Source: CAD feature listing. Evaluate the final solid. Frame: model axes, mm. Face numbers are marked on the shaded views. A direction names the side the tool comes from. Give positions to 0.01 mm unless a question says otherwise; leave off trailing zeros. Order: outer loops, then holes, each group sorted by start corner. A loop starts at its lowest first (then second) coordinate and runs counter-clockwise, first axis right, second up.
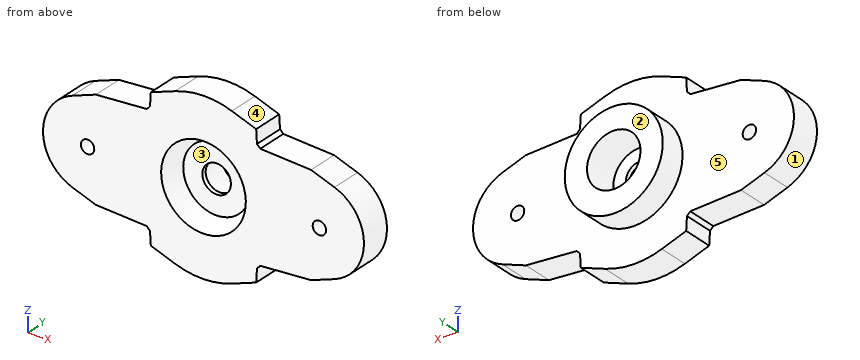
from build123d import *

# Parameters (mm, degrees)
SKETCH1_R           = 5.5
SKETCH1_R_2         = 3
BOSS_EXTRUDE1_DEPTH = 6.5
SKETCH2_R           = 3
BOSS_EXTRUDE2_DEPTH = 3.5
SKETCH4_R           = 3
SKETCH4_R_2         = 1.6
BOSS_EXTRUDE3_DEPTH = 2.5
SKETCH3_R           = 3.75
CUT_EXTRUDE2_DEPTH  = 2
CHAMFER1_SIZE2      = 2
CHAMFER1_SIZE       = 1
SKETCH5_R           = 0.75
CUT_EXTRUDE4_DEPTH  = 40.430318284
SKETCH6_OUTSIDE_W   = 72.61
SKETCH6_OUTSIDE_H   = 72.61
CUT_EXTRUDE5_DEPTH  = 40.430318284


with BuildPart() as part:
    # Sketch1 → Boss-Extrude1 (new body)
    with BuildSketch(Plane(origin=(0, 0, 0), x_dir=(1, 0, 0), z_dir=(0, 1, 0))):
        with Locations(Location((0, 0, 0), (0, 0, 90))):
            Circle(SKETCH1_R)
        with Locations(Location((0, 0, 0), (0, 0, 90))):
            Circle(SKETCH1_R_2, mode=Mode.SUBTRACT)
    extrude(amount=BOSS_EXTRUDE1_DEPTH)

    # Sketch2 → Boss-Extrude2 (add)
    with BuildSketch(Plane(origin=(0, 0, 0), x_dir=(1, 0, 0), z_dir=(0, 1, 0))):
        with BuildLine():
            Line((-6, 6.368869601), (-4.990599203, 22.806463037))
            ThreePointArc((-4.990599203, 22.806463037), (0, 27.5), (4.990599203, 22.806463037))
            Line((4.990599203, 22.806463037), (6, 6.368869601))
            ThreePointArc((6, 6.368869601), (6.187184335, 6.187184335), (6.368869601, 6))
            Line((6.368869601, 6), (22.806463037, 4.990599203))
            ThreePointArc((22.806463037, 4.990599203), (27.5, 0), (22.806463037, -4.990599203))
            Line((22.806463037, -4.990599203), (6.368869601, -6))
            ThreePointArc((6.368869601, -6), (6.187184335, -6.187184335), (6, -6.368869601))
            Line((6, -6.368869601), (4.990599203, -22.806463037))
            ThreePointArc((4.990599203, -22.806463037), (0, -27.5), (-4.990599203, -22.806463037))
            Line((-4.990599203, -22.806463037), (-6, -6.368869601))
            ThreePointArc((-6, -6.368869601), (-6.187184335, -6.187184335), (-6.368869601, -6))
            Line((-6.368869601, -6), (-22.806463037, -4.990599203))
            ThreePointArc((-22.806463037, -4.990599203), (-27.5, 0), (-22.806463037, 4.990599203))
            Line((-22.806463037, 4.990599203), (-6.368869601, 6))
            ThreePointArc((-6.368869601, 6), (-6.187184335, 6.187184335), (-6, 6.368869601))
        make_face()
        with Locations(Location((0, 0, 0), (0, 0, 90))):
            Circle(SKETCH2_R, mode=Mode.SUBTRACT)
    extrude(amount=BOSS_EXTRUDE2_DEPTH)

    # Sketch4 → Boss-Extrude3 (add)
    with BuildSketch(Plane(origin=(0, 0, 0), x_dir=(1, 0, 0), z_dir=(0, 1, 0))):
        with Locations(Location((0, 0, 0), (0, 0, 90))):
            Circle(SKETCH4_R)
        with Locations(Location((0, 0, 0), (0, 0, 270))):
            Circle(SKETCH4_R_2, mode=Mode.SUBTRACT)
    extrude(amount=BOSS_EXTRUDE3_DEPTH)

    # Sketch3 → Cut-Extrude2 (cut)
    with BuildSketch(Plane(origin=(0, 0, 0), x_dir=(1, 0, 0), z_dir=(0, 1, 0))):
        with Locations(Location((0, 0, 0), (0, 0, 270))):
            Circle(SKETCH3_R)
    extrude(amount=CUT_EXTRUDE2_DEPTH, mode=Mode.SUBTRACT)

    # Chamfer1
    chamfer1_edges = [part.edges().sort_by_distance(p)[0] for p in [
        (0, 0, -3.75),
    ]]
    chamfer1_side = [part.faces().sort_by_distance(p)[0] for p in [
        (0, 0, -3.77),
    ]]
    chamfer(chamfer1_edges, length=CHAMFER1_SIZE - 0.0001, length2=CHAMFER1_SIZE2 - 0.0001, reference=chamfer1_side[0])  # a hair under: the kernel refuses the full size

    # Sketch5 → Cut-Extrude4 (cut, through all)
    with BuildSketch(Plane(origin=(0, 0, 0), x_dir=(1, 0, 0), z_dir=(0, 1, 0))):
        with Locations(Location((0, 15, 0), (0, 0, 90))):
            Circle(SKETCH5_R)
        with Locations(Location((0, 21, 0), (0, 0, 90))):
            Circle(SKETCH5_R)
        with Locations(Location((13, 0, 0), (0, 0, 90))):
            Circle(SKETCH5_R)
        with Locations(Location((19, 0, 0), (0, 0, 90))):
            Circle(SKETCH5_R)
        with Locations(Location((25, 0, 0), (0, 0, 90))):
            Circle(SKETCH5_R)
        with Locations(Location((0, -21, 0), (0, 0, 90))):
            Circle(SKETCH5_R)
        with Locations(Location((0, -15, 0), (0, 0, 90))):
            Circle(SKETCH5_R)
        with Locations(Location((-13, 0, 0), (0, 0, 90))):
            Circle(SKETCH5_R)
        with Locations(Location((-19, 0, 0), (0, 0, 90))):
            Circle(SKETCH5_R)
        with Locations(Location((-25, 0, 0), (0, 0, 90))):
            Circle(SKETCH5_R)
    extrude(amount=CUT_EXTRUDE4_DEPTH, mode=Mode.SUBTRACT)

    # Sketch6 outside → Cut-Extrude5 (cut, through all)
    with BuildSketch(Plane.XZ):
        Rectangle(SKETCH6_OUTSIDE_W, SKETCH6_OUTSIDE_H)
        with BuildLine():
            Line((3.181538462, -8.845214131), (14.692307692, -4.704901133))
            ThreePointArc((14.692307692, -4.704901133), (18, 0), (14.692307692, 4.704901133))
            Line((14.692307692, 4.704901133), (3.181538462, 8.845214131))
            ThreePointArc((3.181538462, 8.845214131), (0, 9.4), (-3.181538462, 8.845214131))
            Line((-3.181538462, 8.845214131), (-14.692307692, 4.704901133))
            ThreePointArc((-14.692307692, 4.704901133), (-18, 0), (-14.692307692, -4.704901133))
            Line((-14.692307692, -4.704901133), (-3.181538462, -8.845214131))
            ThreePointArc((-3.181538462, -8.845214131), (0, -9.4), (3.181538462, -8.845214131))
        make_face(mode=Mode.SUBTRACT)
    extrude(amount=-CUT_EXTRUDE5_DEPTH, mode=Mode.SUBTRACT)


solid = part.part
1) Reachability of the marked faces 4 and 5 from +Z, -Z, +X, -X, +Y, -Y: full face, straight path, thin tool, end or side. Return the list, or none.
Checks:
face 4: +Z, +X, +Y, -Y
face 5: +Y
2) Pull-direction query (X, two-part tool) for the marked faces 1, 2 and 3; classes: +X half, -X half, draft (parallel to the pull), parting line (faces both ways), or undercut.
Checks:
face 1: -X half
face 2: draft
face 3: undercut
3) Ray query, L1, parallel to X at y = 2.75, z = 0.5; L2, parallel to Y at x = -9, z = 0.5; L3, parallel to Z at x = 1, y = 6.25. Return the intervals inside material, ascending.
Checks:
L1: x = -17.97 to -13.56, -12.44 to -2.96, 2.96 to 12.44, 13.56 to 17.97
L2: y = 0 to 3.5
L3: z = -5.41 to -2.83, 2.83 to 5.41
4) First-contact query: pin 1 Ø3 at (y, z) = (6, 0.5) entering from -X; pin 2 Ø0.9 at (x, z) = (13, 0) entering from -Y; pin 3 Ø3 at (x, z) = (6, 7.5) entering from +Y; pin 4 Ø3.5 at (x, z) = (0, 0) entering from -Y. Flat tips, straight axial feed; report the tip coordinate or a pass-through.
Checks:
pin 1: stops at x = -5.5
pin 2: passes through
pin 3: stops at y = 3.5
pin 4: stops at y = 2
5) Section query B-B on z = 0. State how many separate pieces and enclosed holes the cut face has, and give its area (3 significant figures).
Checks:
separate pieces: 4
enclosed holes: 0
area: 106 mm2
6) Section query C-C on y = 0.5. Output: boundary loops of the cut face in (x, z), and give its area (3 significant figures).
Checks:
outline: (-14.69, -4.7) - (-12.06, -5.65) - (-6.37, -6) arc R8.75 ccw to (-6, -6.37) - (-5.91, -7.86) - (-3.18, -8.85) arc R9.4 ccw to (3.18, -8.85) - (5.91, -7.86) - (6, -6.37) arc R8.75 ccw to (6.37, -6) - (12.06, -5.65) - (14.69, -4.7) arc R5 ccw to (14.69, 4.7) - (12.06, 5.65) - (6.37, 6) arc R8.75 ccw to (6, 6.37) - (5.91, 7.86) - (3.18, 8.85) arc R9.4 ccw to (-3.18, 8.85) - (-5.91, 7.86) - (-6, 6.37) arc R8.75 ccw to (-6.37, 6) - (-12.06, 5.65) - (-14.69, 4.7) arc R5 ccw to start; hole circle Ø1.5 at (-13, 0); hole circle Ø9 at (0, 0); hole circle Ø1.5 at (13, 0)
area: 386 mm2
7) Section query D-D on y = 5.25. Output: boundary loops of the cut face in (x, z), and give its area (3 significant figures).
Checks:
outline: circle Ø11 at (0, 0); hole circle Ø6 at (0, 0)
area: 66.8 mm2
